For this review, take the finished solid that the model builds, in its own axes (mm). A direction names the side the tool comes from. Coordinates: 2 decimals unless noted, no trailing zeros. Loops run counter-clockwise (first coordinate to the right, second up) from the corner with the lowest first, then second, coordinate; pieces in that order, holes last. Notation, with made-up numbers: (-36.5, -3.5) -> (-30.5, -3.5) arc R24 cw to (-30.5, 30.5) -> close; hole circle Ø7 at (75, 9.25). An arc over 180 degrees is marked (long way). Answer in a Markdown table with one row per item.
from build123d import *

# Parameters (mm, degrees)
SKETCH1_W           = 195
SKETCH1_H           = 67
BOSS_EXTRUDE1_DEPTH = 25.4
CUT_EXTRUDE1_DEPTH  = 107.177492907
CUT_EXTRUDE2_DEPTH  = 121.997561959
CUT_EXTRUDE3_START  = -13
SKETCH4_W           = 3.612655346
SKETCH4_H           = 3
CUT_EXTRUDE3_DEPTH  = 13
SKETCH6_R           = 2.5
CUT_EXTRUDE4_DEPTH  = 107.177492907
SKETCH7_W           = 37
SKETCH7_H           = 35
CUT_EXTRUDE5_DEPTH  = 1.5
CUT_EXTRUDE6_DEPTH  = 18.5
SKETCH9_R           = 2
BOSS_EXTRUDE2_DEPTH = 11
FILLET1_R           = 10


with BuildPart() as part:
    # Sketch1 → Boss-Extrude1 (new body)
    with BuildSketch(Plane(origin=(0, 0, 0), x_dir=(1, 0, 0), z_dir=(0, 1, 0))):
        Rectangle(SKETCH1_W, SKETCH1_H)
    extrude(amount=BOSS_EXTRUDE1_DEPTH)

    # Sketch2 → Cut-Extrude1 (cut, through all)
    with BuildSketch(Plane.XZ):
        with BuildLine():
            Line((97.5, -3.219751644), (97.5, 33.5))
            Line((97.5, 33.5), (88.5, 33.5))
            ThreePointArc((88.5, 33.5), (95.217186872, 15.683556008), (97.5, -3.219751644))
        make_face()
        with BuildLine():
            Line((97.5, -33.5), (97.5, -3.219751644))
            ThreePointArc((97.5, -3.219751644), (95.985558513, -18.65423771), (91.5, -33.5))
            Line((91.5, -33.5), (97.5, -33.5))
        make_face()
        with BuildLine():
            ThreePointArc((-88, -33.5), (-95.08607052, -15.861694529), (-97.5, 2.992884749))
            Line((-97.5, 2.992884749), (-97.5, -33.5))
            Line((-97.5, -33.5), (-88, -33.5))
        make_face()
        with BuildLine():
            ThreePointArc((-97.5, 2.992884749), (-95.856964648, 18.588830376), (-91, 33.5))
            Line((-91, 33.5), (-97.5, 33.5))
            Line((-97.5, 33.5), (-97.5, 2.992884749))
        make_face()
    extrude(amount=-CUT_EXTRUDE1_DEPTH, mode=Mode.SUBTRACT)

    # Sketch3 → Cut-Extrude2 (cut, through all)
    with BuildSketch(Plane(origin=(0, 0, 33.5), x_dir=(-1, 0, 0), z_dir=(0, 0, -1))):
        Polygon((63.2, 25.4), (63.2, 15), (40.2, 15), (40.2, 11), (-61.8, 11), (-61.8, 15), (-97.5, 15), (-97.5, 25.4), align=None)
    extrude(amount=CUT_EXTRUDE2_DEPTH, mode=Mode.SUBTRACT)

    # Sketch4 → Cut-Extrude3 (cut)
    with BuildSketch(Plane(origin=(0, 25.4, 0), x_dir=(1, 0, 0), z_dir=(0, 1, 0)).offset(CUT_EXTRUDE3_START)):
        with BuildLine():
            Line((-63.2, 30.5), (-63.2, 33.5))
            Line((-63.2, 33.5), (-88, 33.5))
            ThreePointArc((-88, 33.5), (-88.810680862, 32.008999469), (-89.587344654, 30.5))
            Line((-89.587344654, 30.5), (-63.2, 30.5))
        make_face()
        with Locations((-61.393672327, 32)):
            Rectangle(SKETCH4_W, SKETCH4_H)
        with BuildLine():
            Line((-63.2, -33.5), (-63.2, -30.5))
            Line((-63.2, -30.5), (-92.261692194, -30.5))
            ThreePointArc((-92.261692194, -30.5), (-91.647155152, -32.006859002), (-91, -33.5))
            Line((-91, -33.5), (-63.2, -33.5))
        make_face()
        with Locations((-61.393672327, -32)):
            Rectangle(SKETCH4_W, SKETCH4_H)
    extrude(amount=CUT_EXTRUDE3_DEPTH, mode=Mode.SUBTRACT)

    # Sketch6 → Cut-Extrude4 (cut, through all)
    with BuildSketch(Plane.XZ):
        with Locations(Location((-28.1, -9, 0), (0, 0, 270))):
            Circle(SKETCH6_R)
        with Locations(Location((-8.2, -8.3, 0), (0, 0, 270))):
            Circle(SKETCH6_R)
        with Locations(Location((-18.7, 8.7, 0), (0, 0, 270))):
            Circle(SKETCH6_R)
        with Locations(Location((-76.2, 22, 0), (0, 0, 270))):
            Circle(SKETCH6_R)
        with Locations(Location((-78.2, 0.1, 0), (0, 0, 270))):
            Circle(SKETCH6_R)
        with Locations(Location((-73.2, -22.3, 0), (0, 0, 270))):
            Circle(SKETCH6_R)
        with Locations(Location((65.3, -20, 0), (0, 0, 270))):
            Circle(SKETCH6_R)
        with Locations(Location((74.1, -1.7, 0), (0, 0, 270))):
            Circle(SKETCH6_R)
        with Locations(Location((68.3, 21.5, 0), (0, 0, 270))):
            Circle(SKETCH6_R)
    extrude(amount=-CUT_EXTRUDE4_DEPTH, mode=Mode.SUBTRACT)

    # Sketch7 → Cut-Extrude5 (cut)
    with BuildSketch(Plane(origin=(0, 11, 0), x_dir=(1, 0, 0), z_dir=(0, 1, 0))):
        with Locations((5.3, -16)):
            Rectangle(SKETCH7_W, SKETCH7_H)
    extrude(amount=-CUT_EXTRUDE5_DEPTH, mode=Mode.SUBTRACT)

    # Sketch8 → Cut-Extrude6 (cut)
    with BuildSketch(Plane(origin=(0, 25.4, 0), x_dir=(1, 0, 0), z_dir=(0, 1, 0))):
        with BuildLine():
            Line((37.096152423, 33.5), (31.9, 33.5))
            Line((31.9, 33.5), (31.9, 30.5))
            ThreePointArc((31.9, 30.5), (34.9, 31.303847577), (37.096152423, 33.5))
        make_face()
        with BuildLine():
            Line((31.9, 33.5), (26.703847577, 33.5))
            ThreePointArc((26.703847577, 33.5), (28.9, 31.303847577), (31.9, 30.5))
            Line((31.9, 30.5), (31.9, 33.5))
        make_face()
    extrude(amount=-CUT_EXTRUDE6_DEPTH, mode=Mode.SUBTRACT)

    # Sketch9 → Boss-Extrude2 (add)
    with BuildSketch(Plane.XZ):
        with BuildLine():
            Line((88.5, 33.5), (137.200361796, 33.5))
            ThreePointArc((137.200361796, 33.5), (142.769729546, 32.427747228), (147.542861296, 29.364285714))
            ThreePointArc((147.542861296, 29.364285714), (154.743476693, 16.527679502), (153.473750823, 1.864285714))
            ThreePointArc((153.473750823, 1.864285714), (147.953179578, -4.940573023), (139.572717606, -7.5))
            Line((139.572717606, -7.5), (97.384558849, -7.5))
            ThreePointArc((97.384558849, -7.5), (95.698800641, 13.597328658), (88.5, 33.5))
        make_face()
        with Locations(Location((138.3, 5.25, 0), (0, 0, 270))):
            Circle(SKETCH9_R, mode=Mode.SUBTRACT)
        with Locations(Location((138.3, 22.75, 0), (0, 0, 270))):
            Circle(SKETCH9_R, mode=Mode.SUBTRACT)
    extrude(amount=-BOSS_EXTRUDE2_DEPTH)

    # Fillet1
    fillet1_edges = [part.edges().sort_by_distance(p)[0] for p in [
        (97.384558849, 5.5, -7.5),
    ]]
    fillet(fillet1_edges, radius=FILLET1_R)


solid = part.part
Item 1: Take a section at B-B, the plane x = -50. State the section outline as (y, z) points.
Worked answers:
| item | result |
|---|---|
| outline | (0, -33.5) -> (15, -33.5) -> (15, 33.5) -> (0, 33.5) -> close |
Item 2: For L1, parallel to X at y = 6.75, z = -9; L2, parallel to X at y = 12.25, z = 21.5; L3, parallel to X at y = 14.75, z = 0.1, list the stretches that pass through material, from the lowest coordinate up.
Worked answers:
| item | result |
|---|---|
| L1 | -96.53 to -30.6, -25.6 to -10.6, -5.8 to 101.08 |
| L2 | -95.18 to -78.65, -73.75 to -40.2, 61.8 to 65.8, 70.8 to 93.55 |
| L3 | -97.44 to -80.7, -75.7 to -40.2, 61.8 to 72.37, 75.83 to 97.43 |
Item 3: Insertion check: pin 1 (15 mm diameter, centred on x = 121.5, z = 18.5, fed in from +Y); pin 2 (2 mm diameter, centred on y = 13, z = 21, fed in from +X); pin 3 (6 mm diameter, centred on y = 5.5, z = -13.5, fed in from +X); pin 4 (4.5 mm diameter, centred on x = 68.3, z = 21.5, fed in from -Y). Each pin has a flat end and moves straight along its axis. Give the tip position at first contact, or say it passes through.
Worked answers:
| item | result |
|---|---|
| pin 1 | y = 11 |
| pin 2 | x = 94.03 |
| pin 3 | x = 99.21 |
| pin 4 | through |
Item 4: Take a section at C-C, the plane x = 103. State the section outline as (y, z) points, and give its area (3 significant figures).
Worked answers:
| item | result |
|---|---|
| outline | (0, -8.08) -> (11, -8.08) -> (11, 33.5) -> (0, 33.5) -> close |
| area | 457 mm² |
Item 5: The part is to be moulded in two halves that separate along X. For faces 1 (the cylindrical face through (140.283, 5.423, 23.01)), 2 (the flat face through (-63.2, 20, 0)), 3 (the flat face through (22, 6, 33.5)), 4 (the flat face through (-40.2, 13, 0)), say which applies: +X half, -X half, draft (parallel to the pull), parting line (faces both ways), or undercut.
Worked answers:
| item | result |
|---|---|
| face 1 | undercut |
| face 2 | +X half |
| face 3 | draft |
| face 4 | undercut |
Item 6: Take a section at A-A, the plane x = -18.7. State the section outline as (y, z) points, and give its area (3 significant figures).
Worked answers:
| item | result |
|---|---|
| outline | (0, -33.5) -> (11, -33.5) -> (11, 6.2) -> (0, 6.2) -> close; (0, 11.2) -> (11, 11.2) -> (11, 33.5) -> (0, 33.5) -> close |
| area | 682 mm² |
Item 7: For faces 5 (the flat face through (123, 5, -7.5)), 6 (the cylindrical face through (154.7, 5.42, 16.73)), 7 (the flat face through (79, 15, 0)), list the 3-axis set-ups (+Z, -Z, +X, -X, +Y, -Y) from which the entire face can be reached by the end or side of a thin tool; tool diameter is ignored.
Worked answers:
| item | result |
|---|---|
| face 5 | -Z, +X, +Y, -Y |
| face 6 | +X, +Y, -Y |
| face 7 | +Z, -Z, +X, +Y |
